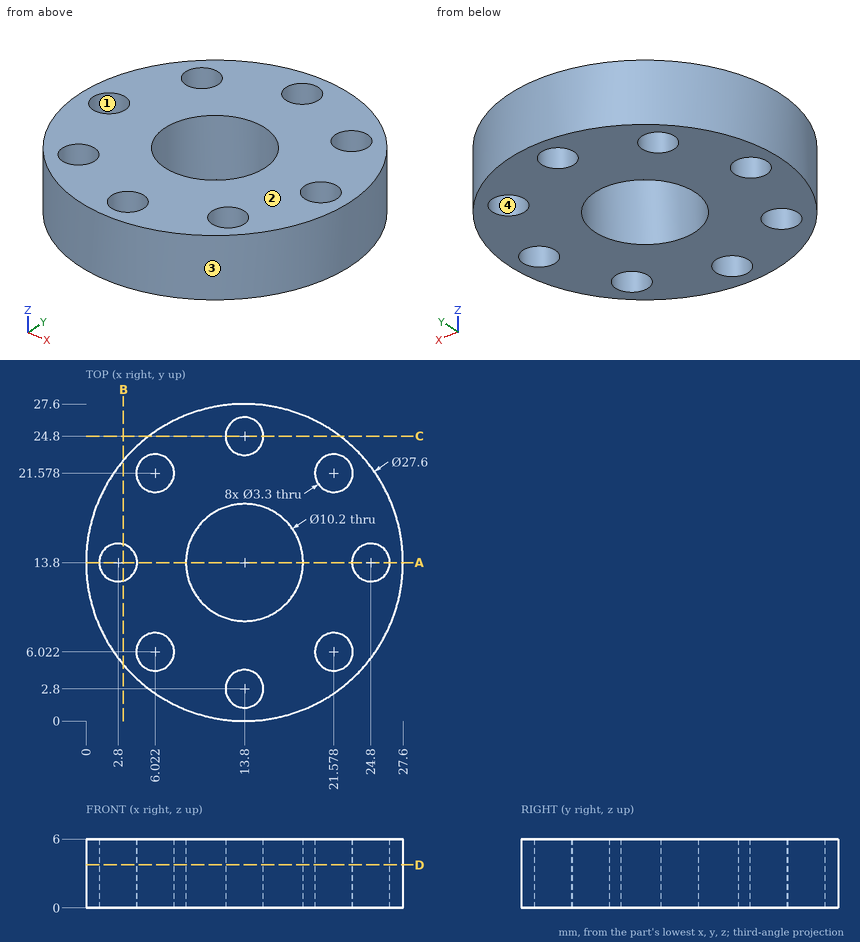
Here's the drawing with two shaded views (mm, measured from the low corner). I have some questions. Give positions to 0.01 mm unless a question says otherwise; leave off trailing zeros. Order: outer loops, then holes, each group sorted by start corner. A loop starts at its lowest first (then second) coordinate and runs counter-clockwise, first axis right, second up. Notation, with made-up numbers: M -17,-24.75 L 29,-24.75 A7 ccw 29,-11.75 Z; hole C -39,-40 d3. An arc over 180 degrees is marked long. One line per item, written item: value.
1) We'd pull the mould along Y, two halves only. Please class the marked faces 1, 2, 3 and 4: released by +Y, released by -Y, zero draft, split by the parting line, or undercut.
Answer sheet:
face 1: undercut
face 2: zero draft
face 3: split by the parting line
face 4: undercut
2) Please list where these lines run through material, in increasing order: line 1 along Y through (x, z) = (24.75, 0.3); line 2 along X through (y, z) = (4, 3.95) (1 decimal); line 3 along X through (y, z) = (24, 0.6) (1 decimal).
Answer sheet:
line 1: y = 5.4 to 12.15, 15.45 to 22.2
line 2: x = 4.1 to 12.7, 14.9 to 23.5
line 3: x = 4.5 to 12.4, 15.2 to 23.1
3) I want a section at B-B, the plane x = 3.25. List the corners of the cut face in (y, z) for me.
Answer sheet:
outline: M 4.9,0 L 12.21,0 L 12.21,6 L 4.9,6 Z; M 15.39,0 L 22.7,0 L 22.7,6 L 15.39,6 Z
4) I want a section at C-C, the plane y = 24.8. List the corners of the cut face in (x, z) for me, plus the area to 3 significant figures.
Answer sheet:
outline: M 5.47,0 L 12.15,0 L 12.15,6 L 5.47,6 Z; M 15.45,0 L 22.13,0 L 22.13,6 L 15.45,6 Z
area: 80.2 mm^2
5) I want a section at A-A, the plane y = 13.8. List the corners of the cut face in (x, z) for me.
Answer sheet:
outline: M 0,0 L 1.15,0 L 1.15,6 L 0,6 Z; M 4.45,0 L 8.7,0 L 8.7,6 L 4.45,6 Z; M 18.9,0 L 23.15,0 L 23.15,6 L 18.9,6 Z; M 26.45,0 L 27.6,0 L 27.6,6 L 26.45,6 Z
6) I want a section at D-D, the plane z = 3.75. Count the separate pieces of the cut face and the enclosed holes in it, plus the area to 3 significant figures.
Answer sheet:
separate pieces: 1
enclosed holes: 9
area: 448 mm^2
7) For P1, Ø2.5, axis at x = 2.8, y = 13.8, coming from the -Z side; P2, Ø3, axis at x = 8.5, z = 1, coming from the +Y side; P3, Ø5.5, axis at x = 21.58, y = 21.58, coming from the +Z side; P4, Ø3, axis at y = 9, z = 5, coming from the -X side, each with a flat end and sliding along its axis, tell me the tip position at first contact or that it passes through.
Answer sheet:
P1: passes through
P2: stops at y = 27.07
P3: stops at z = 6
P4: stops at x = 0.4
